```python
from build123d import *

# Parameters (mm, degrees)
SKETCH1_W               = 22.606
SKETCH1_H               = 10.033
BOSS_EXTRUDE1_DEPTH     = 0.5715
CUT_EXTRUDE1_DEPTH      = 25.758812047
CUT_EXTRUDE1_DEPTH_BACK = 25.758812047
SKETCH2_R               = 0.9906
SKETCH3_W               = 23.2918
SKETCH3_H               = 2.3876
BOSS_EXTRUDE2_DEPTH     = 8.636
SKETCH4_W               = 3.429
SKETCH4_H               = 2.54
BOSS_EXTRUDE3_DEPTH     = 1.143
LPATTERN1_COUNT         = 3
LPATTERN1_PITCH         = 8.001
MIRROR4_COPY_1_SKETCH_W = 3.429
MIRROR4_COPY_1_SKETCH_H = 2.54
MIRROR4_COPY_1_DEPTH    = 1.143
MIRROR4_COPY_2_SKETCH_W = 3.429
MIRROR4_COPY_2_SKETCH_H = 2.54
MIRROR4_COPY_2_DEPTH    = 1.143


with BuildPart() as part:
    # Sketch1 → Boss-Extrude1 (new, symmetric)
    with BuildSketch(Plane(origin=(0, 0, 0), x_dir=(1, 0, 0), z_dir=(0, 1, 0))):
        with Locations((-11.303, 5.0165)):
            Rectangle(SKETCH1_W, SKETCH1_H)
    boss_extrude1 = extrude(amount=BOSS_EXTRUDE1_DEPTH, both=True)

    # Mirror1: Boss-Extrude1 across plane
    add(boss_extrude1.mirror(Plane(origin=(0, 0.5715, 0), x_dir=(1, 0, 0), z_dir=(0, 0, -1))))

    # Sketch2 → Cut-Extrude1 (cut, two sides: drawn at the far end of the back side and taken through both)
    with BuildSketch(Plane(origin=(0, 0.5715, 0), x_dir=(1, 0, 0), z_dir=(0, 1, 0)).offset(-CUT_EXTRUDE1_DEPTH_BACK)):
        with Locations(Location((-19.84375, 7.61365, 0), (0, 0, 270))):
            Circle(SKETCH2_R)
    extrude(amount=CUT_EXTRUDE1_DEPTH + CUT_EXTRUDE1_DEPTH_BACK, mode=Mode.SUBTRACT)

    # Mirror3: part across plane


with BuildPart() as part_1:
    add(part.part)
    add(part.part.mirror(Plane(origin=(0, 0, 0), x_dir=(0, 0, 1), z_dir=(1, 0, 0))))

    # Sketch3 → Boss-Extrude2 (add)
    with BuildSketch(Plane(origin=(0, 0.5715, 0), x_dir=(1, 0, 0), z_dir=(0, 1, 0))):
        with Locations((0, -8.5852)):
            Rectangle(SKETCH3_W, SKETCH3_H)
    extrude(amount=BOSS_EXTRUDE2_DEPTH)

    # Sketch4 → Boss-Extrude3 (add)
    with BuildSketch(Plane.XZ.offset(0.5715)):
        with Locations((-19.84375, -2.53365)):
            Rectangle(SKETCH4_W, SKETCH4_H)
    boss_extrude3 = extrude(amount=BOSS_EXTRUDE3_DEPTH)

    # LPattern1: Boss-Extrude3 ×3
    with Locations(*[(i * LPATTERN1_PITCH, 0, 0) for i in range(1, LPATTERN1_COUNT)]):
        add(boss_extrude3)

    # Mirror4: Boss-Extrude3 across plane
    add(boss_extrude3.mirror(Plane(origin=(0, 0, 0), x_dir=(0, 0, 1), z_dir=(1, 0, 0))))

    # Mirror4 copy 1 sketch → Mirror4 copy 1 (add)
    with BuildSketch(Plane(origin=(-8.001, -0.5715, 0), x_dir=(-1, 0, 0), z_dir=(0, -1, 0))):
        with Locations((-19.84375, 2.53365)):
            Rectangle(MIRROR4_COPY_1_SKETCH_W, MIRROR4_COPY_1_SKETCH_H)
    extrude(amount=MIRROR4_COPY_1_DEPTH)

    # Mirror4 copy 2 sketch → Mirror4 copy 2 (add)
    with BuildSketch(Plane(origin=(-16.002, -0.5715, 0), x_dir=(-1, 0, 0), z_dir=(0, -1, 0))):
        with Locations((-19.84375, 2.53365)):
            Rectangle(MIRROR4_COPY_2_SKETCH_W, MIRROR4_COPY_2_SKETCH_H)
    extrude(amount=MIRROR4_COPY_2_DEPTH)


solid = part_1.part
```
The model under review builds one solid part; all positions refer to its coordinate system, in mm. A direction names the side the tool comes from. Coordinates: 2 decimals unless noted, no trailing zeros. Write each loop counter-clockwise with the first axis right and the second up, starting at its lowest first coordinate (ties: lowest second). Pieces come first, ordered by that corner, then holes. Notation, with made-up numbers: (32.25, 57) -> (70.25, 57) arc R27 ccw to (70.25, 94) -> close; hole circle Ø8 at (76, 31.5). An arc over 180 degrees is marked (long way). One line per item, written item: value. Start each with the question number.
Q1. Add section A-A, the plane x = -7. Give the boundary of the cut face in (y, z).
Q2. For faces 1 (the face through (21.558, -1, -3)), 2 (the face through (4, -1, -3.804)), 3 (the face through (12, -1, -1.264)), 4 (the face through (11.646, 5, 9)), 5 (the face through (13.557, -1, -3)), list the 3-axis set-ups (+Z, -Z, +X, -X, +Y, -Y) from which the entire face can be reached by the end or side of a thin tool; tool diameter is ignored.
Q3. Clearance check with flat-ended pins moving along their axes: P1, Ø0.6, axis at y = -1, z = -3, coming from the -X side; P2, Ø2.5, axis at y = 4.5, z = 8.5, coming from the +X side; P3, Ø0.6, axis at x = 11.5, y = -1, coming from the -Z side; P4, Ø1.3, axis at x = -4.5, y = -1, coming from the +Z side. State where each tip first meets the part, or that it passes through.
Q4. Add section B-B, the plane z = 8. Give the boundary of the cut face in (x, y).
Q5. Add section C-C, the plane z = -7.25. Give the boundary of the cut face in (x, y), then the cut area to 3 significant figures.
Q6. To check wall thickness, follow probe 1 along Z at (x, y) = (18.5, -1); probe 2 along Z at (x, y) = (-20, -0.5); probe 3 along Z at (x, y) = (9, 3). State the ranges of each line that lie inside material, in increasing order.
Q7. The part is to be moulded in two halves that separate along X. For faces 6 (the face through (-20, -1, -1.264)), 7 (the face through (2.127, -1, -3)), 8 (the face through (-21.558, -1, -3)), say which applies: +X half, -X half, draft (parallel to the pull), parting line (faces both ways), or undercut.
Q8. Add section D-D, the plane y = 3.75. Give the boundary of the cut face in (x, z).
Response:
1. outline: (-0.57, -10.03) -> (0.57, -10.03) -> (0.57, 7.39) -> (9.21, 7.39) -> (9.21, 9.78) -> (0.57, 9.78) -> (0.57, 10.03) -> (-0.57, 10.03) -> close
2. face 1: +Z, -Z, +X, -Y
2. face 2: -Z, +X, -X, -Y
2. face 3: +Z, +X, -X, -Y
2. face 4: +Z, -Z, +X, +Y
2. face 5: +Z, -Z, -Y
3. P1: x = -21.56
3. P2: x = 11.65
3. P3: z = -3.8
3. P4: z = 10.03
4. outline: (-22.61, -0.57) -> (22.61, -0.57) -> (22.61, 0.57) -> (11.65, 0.57) -> (11.65, 9.21) -> (-11.65, 9.21) -> (-11.65, 0.57) -> (-22.61, 0.57) -> close
5. outline: (-22.61, -0.57) -> (-20.77, -0.57) -> (-20.77, 0.57) -> (-22.61, 0.57) -> close; (-18.92, -0.57) -> (18.92, -0.57) -> (18.92, 0.57) -> (-18.92, 0.57) -> close; (20.77, -0.57) -> (22.61, -0.57) -> (22.61, 0.57) -> (20.77, 0.57) -> close
5. area: 47.5 mm²
6. probe 1: -3.8 to -1.26
6. probe 2: -10.03 to -8.59, -6.64 to 10.03
6. probe 3: 7.39 to 9.78
7. face 6: draft
7. face 7: undercut
7. face 8: -X half
8. outline: (-11.65, 7.39) -> (11.65, 7.39) -> (11.65, 9.78) -> (-11.65, 9.78) -> close
